from build123d import *

# Parameters (mm, degrees)
F1_DEPTH = 0.61


with BuildPart() as f1:
    # F0 (on Front) → F1 (new body)
    with BuildSketch(Plane.XZ):
        with BuildLine():
            Line((-30, 0), (0, 0))
            Line((0, 0), (30.000002, 0))
            Line((30.000002, 0), (15.5, 20.689656))
            Line((15.5, 20.689656), (4.5, 20.689656))
            Line((4.5, 20.689656), (4.5, 18.689656))
            ThreePointArc((4.5, 18.689656), (3, 17.189656), (1.5, 18.689656))
            Line((1.5, 18.689656), (1.5, 20.689656))
            Line((1.5, 20.689656), (0, 20.689656))
            Line((0, 20.689656), (-1.5, 20.689656))
            Line((-1.5, 20.689656), (-1.5, 18.689656))
            ThreePointArc((-1.5, 18.689656), (-3, 17.189656), (-4.5, 18.689656))
            Line((-4.5, 18.689656), (-4.5, 20.689656))
            Line((-4.5, 20.689656), (-15.5, 20.689656))
            Line((-15.5, 20.689656), (-30, 0))
        make_face()
    extrude(amount=F1_DEPTH)


solid = f1.part
The listing builds one solid part. Answer for the finished solid, in the listing's coordinates (mm). Give positions to 0.01 mm unless a question says otherwise; leave off trailing zeros. Loops run counter-clockwise (first coordinate to the right, second up) from the corner with the lowest first, then second, coordinate; pieces in that order, holes last.
Item 1: This flat-tipped pin is pushed along its axis until it touches: pin 1 Ø12 at (x, z) = (-1, 13) entering from +Y. Where does it stop, or does it pass through?
Derived:
pin 1: stops at y = 0
Item 2: A cutting plane is placed at C-C (x = -3). Give the vertices of the cut face in (y, z).
Derived:
outline: (-0.61, 0) - (0, 0) - (0, 17.19) - (-0.61, 17.19) - close
Item 3: A cutting plane is placed at A-A (y = -0.5). Give the vertices of the cut face in (x, z), then the cut area to 3 significant figures.
Derived:
outline: (-30, 0) - (30, 0) - (15.5, 20.69) - (4.5, 20.69) - (4.5, 18.69) arc R1.5 cw to (1.5, 18.69) - (1.5, 20.69) - (-1.5, 20.69) - (-1.5, 18.69) arc R1.5 cw to (-4.5, 18.69) - (-4.5, 20.69) - (-15.5, 20.69) - close
area: 922 mm2
Item 4: Find the intervals of material crossed by line 1 along X through (y, z) = (-0.25, 18.25); line 2 along X through (y, z) = (-0.3, 19); line 3 along X through (y, z) = (-0.15, 13.75), in increasing order.
Derived:
line 1: x = -17.21 to -4.43, -1.57 to 1.57, 4.43 to 17.21
line 2: x = -16.68 to -4.5, -1.5 to 1.5, 4.5 to 16.68
line 3: x = -20.36 to 20.36
Item 5: A cutting plane is placed at B-B (z = 12). Give the vertices of the cut face in (x, y), then the cut area to 3 significant figures.
Derived:
outline: (-21.59, -0.61) - (21.59, -0.61) - (21.59, 0) - (-21.59, 0) - close
area: 26.3 mm2
